```python
from build123d import *

# Parameters (mm, degrees)
SKETCH1_W           = 50.8
SKETCH1_H           = 50.8
SKETCH1_W_2         = 47.625
SKETCH1_H_2         = 47.625
BOSS_EXTRUDE1_DEPTH = 2260.6
SKETCH3_R           = 2.38125
CUT_EXTRUDE2_DEPTH  = 51.8
LPATTERN2_COUNT     = 11
LPATTERN2_PITCH     = 215.9
SKETCH4_R           = 2.38125
CUT_EXTRUDE3_DEPTH  = 50.8
LPATTERN3_COUNT     = 4
LPATTERN3_PITCH     = 635
SKETCH5_R           = 4.445
CUT_EXTRUDE4_DEPTH  = 51.8


with BuildPart() as part:
    # Sketch1 → Boss-Extrude1 (new body)
    with BuildSketch(Plane(origin=(0, 0, 0), x_dir=(0, 0, -1), z_dir=(1, 0, 0))):
        with Locations((25.4, 25.4)):
            Rectangle(SKETCH1_W, SKETCH1_H)
        with Locations((25.4, 25.4)):
            Rectangle(SKETCH1_W_2, SKETCH1_H_2, mode=Mode.SUBTRACT)
    extrude(amount=BOSS_EXTRUDE1_DEPTH)

    # Sketch3 → Cut-Extrude2 (cut, through all)
    with BuildSketch(Plane(origin=(0, 0, -50.8), x_dir=(-1, 0, 0), z_dir=(0, 0, -1))):
        with Locations((-50.8, 25.4)):
            Circle(SKETCH3_R)
    cut_extrude2 = extrude(amount=-CUT_EXTRUDE2_DEPTH, mode=Mode.SUBTRACT)

    # LPattern2: Cut-Extrude2 ×11
    with Locations(*[(i * LPATTERN2_PITCH, 0, 0) for i in range(1, LPATTERN2_COUNT)]):
        add(cut_extrude2, mode=Mode.SUBTRACT)

    # Sketch4 → Cut-Extrude3 (cut)
    with BuildSketch(Plane.XZ):
        with Locations((177.8, -25.4)):
            Circle(SKETCH4_R)
    cut_extrude3 = extrude(amount=-CUT_EXTRUDE3_DEPTH, mode=Mode.SUBTRACT)

    # LPattern3: Cut-Extrude3 ×4
    with Locations(*[(i * LPATTERN3_PITCH, 0, 0) for i in range(1, LPATTERN3_COUNT)]):
        add(cut_extrude3, mode=Mode.SUBTRACT)

    # Sketch5 → Cut-Extrude4 (cut, through all)
    with BuildSketch(Plane.XZ):
        with Locations((1263.65, -25.4)):
            Circle(SKETCH5_R)
    extrude(amount=-CUT_EXTRUDE4_DEPTH, mode=Mode.SUBTRACT)


solid = part.part
```
Can you work these out from the model? Positions are in its coordinate system, mm. A direction names the side the tool comes from. Coordinates: 2 decimals unless noted, no trailing zeros. Loops run counter-clockwise (first coordinate to the right, second up) from the corner with the lowest first, then second, coordinate; pieces in that order, holes last. Notation, with made-up numbers: M -38.5,25.25 L -3.5,25.25 A22 cw -3.5,51.25 Z; hole C -31.5,23 d7. An arc over 180 degrees is marked long. Put each result on its own line as item: value. Start each with the question number.
(1) Which directions (+Z, -Z, +X, -X, +Y, -Y) give clear straight access to the entire face, cutting with the end or side of a thin tool? Please do faces 4 (the face through (0, 1, -23)), 5 (the face through (1114, 49.212, -25)).
(2) We'd pull the mould along Y, two halves only. Please class faces 1 (the face through (1114, 25, -49.212)), 2 (the face through (1114, 25, 0)), 3 (the face through (1114, 50.8, -25)): +Y half, -Y half, draft (parallel to the pull), parting line (faces both ways), or undercut.
(3) I need wall thicknesses on probe 1 along Y at (x, z) = (1130, -49); probe 2 along Y at (x, z) = (1346.2, -0.35); probe 3 along Z at (x, y) = (1420, 6). Which ranges of each line are inside material? Lowest first, please.
(4) Imagine slicing it at B-B on y = 39.5. List the corners of the cut face in (x, z) for me.
(5) Imagine slicing it at A-A on z = -38. List the corners of the cut face in (x, y) for me.
(6) Will this pin go through, and if not, where does the flat tip stop? pin 1 Ø5.5 at (x, z) = (1263.65, -25.4) entering from -Y.
(7) Imagine slicing it at C-C on x = 1026. List the corners of the cut face in (y, z) for me.
Worked answers:
1. face 4: +Z, -Z, -X, +Y, -Y
1. face 5: +X, -X
2. face 1: undercut
2. face 2: draft
2. face 3: +Y half
3. probe 1: y = 0 to 1.59, 49.21 to 50.8
3. probe 2: y = 0 to 23.02, 27.78 to 50.8
3. probe 3: z = -50.8 to -49.21, -1.59 to 0
4. outline: M 0,-50.8 L 2260.6,-50.8 L 2260.6,-49.21 L 0,-49.21 Z; M 0,-1.59 L 2260.6,-1.59 L 2260.6,0 L 0,0 Z
5. outline: M 0,0 L 2260.6,0 L 2260.6,1.59 L 0,1.59 Z; M 0,49.21 L 2260.6,49.21 L 2260.6,50.8 L 0,50.8 Z
6. pin 1: passes through
7. outline: M 0,-50.8 L 50.8,-50.8 L 50.8,0 L 0,0 Z; hole M 1.59,-49.21 L 49.21,-49.21 L 49.21,-1.59 L 1.59,-1.59 Z
